The model under review builds one solid part; all positions refer to its coordinate system, in mm. A direction names the side the tool comes from. Round coordinates to 2 decimals unless told otherwise and drop trailing zeros. Order: outer loops, then holes, each group sorted by start corner. A loop starts at its lowest first (then second) coordinate and runs counter-clockwise, first axis right, second up.
```python
from build123d import *
from OCP.BRepFilletAPI import BRepFilletAPI_MakeChamfer

# Parameters (mm, degrees)
SKETCH3_R               = 27
BOSS_EXTRUDE1_DEPTH     = 6
BOSS_EXTRUDE2_DEPTH     = 126
SKETCH19_R              = 27
BOSS_EXTRUDE3_DEPTH     = 6
CUT_EXTRUDE5_REACH      = 139.412
SKETCH13_R              = 2.6
CUT_EXTRUDE6_REACH      = 145.185
SKETCH20_R              = 2.6
CUT_EXTRUDE7_REACH      = 145.185
SKETCH21_W              = 10
SKETCH21_H              = 41.952353926
RIB3_REACH              = 145.185
SKETCH18_WALL_W         = 329.601445786
SKETCH18_WALL_H         = 5
CIRPATTERN1_COUNT       = 3
MIRROR2_COPY_1_REACH    = 145.185
MIRROR2_COPY_1_SKETCH_W = 329.601445786
MIRROR2_COPY_1_SKETCH_H = 5
MIRROR2_COPY_2_REACH    = 145.185
MIRROR2_COPY_2_SKETCH_W = 329.601445786
MIRROR2_COPY_2_SKETCH_H = 5
FILLET1_R               = 12
CHAMFER1_SIZE           = 1
CHAMFER1_SIZE2          = 1.732050808
CHAMFER2_SIZE           = 1
CHAMFER3_SIZE           = 0.5


with BuildPart() as part:
    # Sketch3 → Boss-Extrude1 (new body)
    with BuildSketch(Plane(origin=(0, 0, 0), x_dir=(1, 0, 0), z_dir=(0, 1, 0))):
        with Locations(Location((0, 0, 0), (0, 0, 270))):
            Circle(SKETCH3_R)
    extrude(amount=BOSS_EXTRUDE1_DEPTH)

    # Sketch4 → Boss-Extrude2 (add)
    with BuildSketch(Plane(origin=(0, 6, 0), x_dir=(1, 0, 0), z_dir=(0, 1, 0))):
        Polygon((10, -5.773502692), (10, 5.773502692), (0, 11.547005384), (-10, 5.773502692), (-10, -5.773502692), (0, -11.547005384), align=None)
    extrude(amount=BOSS_EXTRUDE2_DEPTH)

    # Sketch19 → Boss-Extrude3 (add)
    with BuildSketch(Plane(origin=(0, 132, 0), x_dir=(1, 0, 0), z_dir=(0, 1, 0))):
        with Locations(Location((0, 0, 0), (0, 0, 270))):
            Circle(SKETCH19_R)
    extrude(amount=BOSS_EXTRUDE3_DEPTH)

    # Sketch13 → Cut-Extrude5 (cut, up to next)
    with BuildSketch(Plane(origin=(0, 6, 0), x_dir=(1, 0, 0), z_dir=(0, 1, 0)), mode=Mode.PRIVATE) as cut_extrude5_sk1:
        with Locations(Location((-19, 0, 0), (0, 0, 270))):
            Circle(SKETCH13_R)
    cut_extrude5_tool1 = extrude(cut_extrude5_sk1.sketch, amount=-CUT_EXTRUDE5_REACH, mode=Mode.PRIVATE) & part.part
    # Sketch13 → Cut-Extrude5 (cut, up to next)
    with BuildSketch(Plane(origin=(0, 6, 0), x_dir=(1, 0, 0), z_dir=(0, 1, 0)), mode=Mode.PRIVATE) as cut_extrude5_sk2:
        with Locations(Location((9.5, 16.454482672, 0), (0, 0, 270))):
            Circle(SKETCH13_R)
    cut_extrude5_tool2 = extrude(cut_extrude5_sk2.sketch, amount=-CUT_EXTRUDE5_REACH, mode=Mode.PRIVATE) & part.part
    # Sketch13 → Cut-Extrude5 (cut, up to next)
    with BuildSketch(Plane(origin=(0, 6, 0), x_dir=(1, 0, 0), z_dir=(0, 1, 0)), mode=Mode.PRIVATE) as cut_extrude5_sk3:
        with Locations(Location((9.5, -16.454482672, 0), (0, 0, 270))):
            Circle(SKETCH13_R)
    cut_extrude5_tool3 = extrude(cut_extrude5_sk3.sketch, amount=-CUT_EXTRUDE5_REACH, mode=Mode.PRIVATE) & part.part
    add(cut_extrude5_tool1.solids().sort_by_distance((-19, 6, 0))[0], mode=Mode.SUBTRACT)
    add(cut_extrude5_tool2.solids().sort_by_distance((9.5, 6, -16.454483))[0], mode=Mode.SUBTRACT)
    add(cut_extrude5_tool3.solids().sort_by_distance((9.5, 6, 16.454483))[0], mode=Mode.SUBTRACT)

    # Sketch20 → Cut-Extrude6 (cut, up to next)
    with BuildSketch(Plane(origin=(0, 138, 0), x_dir=(1, 0, 0), z_dir=(0, 1, 0)), mode=Mode.PRIVATE) as cut_extrude6_sk1:
        with Locations(Location((9.5, 16.454482672, 0), (0, 0, 270))):
            Circle(SKETCH20_R)
    cut_extrude6_tool1 = extrude(cut_extrude6_sk1.sketch, amount=-CUT_EXTRUDE6_REACH, mode=Mode.PRIVATE) & part.part
    # Sketch20 → Cut-Extrude6 (cut, up to next)
    with BuildSketch(Plane(origin=(0, 138, 0), x_dir=(1, 0, 0), z_dir=(0, 1, 0)), mode=Mode.PRIVATE) as cut_extrude6_sk2:
        with Locations(Location((9.5, -16.454482672, 0), (0, 0, 270))):
            Circle(SKETCH20_R)
    cut_extrude6_tool2 = extrude(cut_extrude6_sk2.sketch, amount=-CUT_EXTRUDE6_REACH, mode=Mode.PRIVATE) & part.part
    add(cut_extrude6_tool1.solids().sort_by_distance((9.5, 138, -16.454483))[0], mode=Mode.SUBTRACT)
    add(cut_extrude6_tool2.solids().sort_by_distance((9.5, 138, 16.454483))[0], mode=Mode.SUBTRACT)

    # Sketch21 → Cut-Extrude7 (cut, up to next)
    with BuildSketch(Plane(origin=(0, 138, 0), x_dir=(1, 0, 0), z_dir=(0, 1, 0)), mode=Mode.PRIVATE) as cut_extrude7_sk1:
        with Locations((-22, 0)):
            Rectangle(SKETCH21_W, SKETCH21_H)
    cut_extrude7_tool1 = extrude(cut_extrude7_sk1.sketch, amount=-CUT_EXTRUDE7_REACH, mode=Mode.PRIVATE) & part.part
    add(cut_extrude7_tool1.solids().sort_by_distance((-22, 138, 0))[0], mode=Mode.SUBTRACT)

    # Sketch18 wall → Rib3 (add, up to next)
    with BuildSketch(Plane(origin=(15, 26, 0), x_dir=(0.242535625036, -0.970142500145, 0), z_dir=(0.970142500145, 0.242535625036, 0)), mode=Mode.PRIVATE) as rib3_sk1:
        Rectangle(SKETCH18_WALL_W, SKETCH18_WALL_H)
    rib3_tool1 = extrude(rib3_sk1.sketch, amount=-RIB3_REACH, mode=Mode.PRIVATE) - part.part
    rib3 = rib3_tool1.solids().sort_by_distance((15, 26, 0))[0]
    add(rib3)

    # CirPattern1: Rib3 ×3 about axis
    cirpattern1_axis = Axis((0, 0, 0), (0, 1, 0))
    for i in range(1, CIRPATTERN1_COUNT):
        add(rib3.rotate(cirpattern1_axis, i * 360 / CIRPATTERN1_COUNT))

    # Mirror2: Rib3 across plane
    add(rib3.mirror(Plane.ZX.offset(69)))

    # Mirror2 copy 1 sketch → Mirror2 copy 1 (add, up to next)
    with BuildSketch(Plane(origin=(-7.5, 112, -12.990381057), x_dir=(-0.12126781251799995, 0.970142500145, -0.21004201260391314), z_dir=(-0.4850712500724998, -0.242535625036, -0.8401680504165185)), mode=Mode.PRIVATE) as mirror2_copy_1_sk1:
        Rectangle(MIRROR2_COPY_1_SKETCH_W, MIRROR2_COPY_1_SKETCH_H)
    mirror2_copy_1_tool1 = extrude(mirror2_copy_1_sk1.sketch, amount=-MIRROR2_COPY_1_REACH, mode=Mode.PRIVATE) - part.part
    add(mirror2_copy_1_tool1.solids().sort_by_distance((-7.5, 112, -12.990381057))[0])

    # Mirror2 copy 2 sketch → Mirror2 copy 2 (add, up to next)
    with BuildSketch(Plane(origin=(-7.5, 112, 12.990381057), x_dir=(-0.12126781251800012, 0.970142500145, 0.21004201260391306), z_dir=(-0.48507125007250046, -0.242535625036, 0.8401680504165182)), mode=Mode.PRIVATE) as mirror2_copy_2_sk1:
        Rectangle(MIRROR2_COPY_2_SKETCH_W, MIRROR2_COPY_2_SKETCH_H)
    mirror2_copy_2_tool1 = extrude(mirror2_copy_2_sk1.sketch, amount=-MIRROR2_COPY_2_REACH, mode=Mode.PRIVATE) - part.part
    add(mirror2_copy_2_tool1.solids().sort_by_distance((-7.5, 112, 12.990381057))[0])

    # Fillet1
    fillet1_edges = [part.edges().sort_by_distance(p)[0] for p in [
        (-17, 135, 20.976176963),
        (-17, 135, -20.976176963),
    ]]
    fillet(fillet1_edges, radius=FILLET1_R)

    # Chamfer1: one chamfer whose edges measure the first distance from different faces: ONE call of the kernel's chamfer builder (chamfer() names one face for all edges)
    chamfer1_edges_1 = [part.edges().sort_by_distance(p)[0] for p in [
        (10, 132, 4.136751346),
        (5, 132, -8.660254038),
        (-1.417468245, 132, -10.728629711),
        (-10, 132, 0),
        (-8.582531755, 132, 6.591878365),
        (10, 132, -4.136751346),
        (-1.417468245, 132, 10.728629711),
        (-8.582531755, 132, -6.591878365),
        (5, 132, 8.660254038),
    ]]
    chamfer1_side_1 = [part.faces().sort_by_distance(p)[0] for p in [
        (26.303437009, 132, 0),
    ]]
    chamfer1_edges_2 = [part.edges().sort_by_distance(p)[0] for p in [
        (-1.417468245, 6, 10.728629711),
        (-8.582531755, 6, -6.591878365),
        (10, 6, -4.136751346),
        (5, 6, 8.660254038),
        (10, 6, 4.136751346),
        (5, 6, -8.660254038),
        (-1.417468245, 6, -10.728629711),
        (-10, 6, 0),
        (-8.582531755, 6, 6.591878365),
    ]]
    chamfer1_side_2 = [part.faces().sort_by_distance(p)[0] for p in [
        (0, 6, -26.236324676),
    ]]
    chamfer1 = BRepFilletAPI_MakeChamfer(part.part.solid().wrapped)
    for e in chamfer1_edges_1:
        chamfer1.Add(CHAMFER1_SIZE, CHAMFER1_SIZE2, e.wrapped, chamfer1_side_1[0].wrapped)  # the first distance lies on this face
    for e in chamfer1_edges_2:
        chamfer1.Add(CHAMFER1_SIZE, CHAMFER1_SIZE2, e.wrapped, chamfer1_side_2[0].wrapped)  # the first distance lies on this face
    add(Compound.cast(chamfer1.Shape()), mode=Mode.REPLACE)

    # Chamfer2
    chamfer2_edges = [part.edges().sort_by_distance(p)[0] for p in [
        (0, 0, -27),
        (-17, 138, 0),
        (-17, 132, 0),
        (27, 132, 0),
        (-14.797958971, 132, 21.070338854),
        (-14.797958971, 132, -21.070338854),
        (27, 138, 0),
        (-14.797958971, 138, 21.070338854),
        (-14.797958971, 138, -21.070338854),
        (0, 6, -27),
    ]]
    chamfer(chamfer2_edges, length=CHAMFER2_SIZE)

    # Chamfer3
    chamfer3_edges = [part.edges().sort_by_distance(p)[0] for p in [
        (-19, 6, -2.6),
        (-19, 0, -2.6),
        (9.5, 6, -19.054482672),
        (9.5, 0, -19.054482672),
        (9.5, 6, 13.854482672),
        (9.5, 0, 13.854482672),
        (9.5, 132, -19.054482672),
        (9.5, 138, -19.054482672),
        (9.5, 132, 13.854482672),
        (9.5, 138, 13.854482672),
    ]]
    chamfer(chamfer3_edges, length=CHAMFER3_SIZE)


solid = part.part
```
(1) For faces 1 (the flat face through (13, 21, -2.5)), 2 (the flat face through (15, 132, 5)), 3 (the flat face through (-4.136, 20.976, 12.164)), 4 (the flat face through (13, 117, 2.5)), 5 (the flat face through (-9.1, 131.12, 6.86)), list the 3-axis set-ups (+Z, -Z, +X, -X, +Y, -Y) from which the entire face can be reached by the end or side of a thin tool; tool diameter is ignored.
Data:
face 1: -Z, +X
face 2: none
face 3: +Z
face 4: +Z, +X
face 5: -X
(2) Consider section B-B (y = 70). Write out the cut boundary in (x, z), and give its area (3 significant figures).
Data:
outline: (-10, -5.77) - (0, -11.55) - (10, -5.77) - (10, 5.77) - (0, 11.55) - (-10, 5.77) - close
area: 346 mm2
(3) Insertion check: pin 1 (12.5 mm diameter, centred on y = 76, z = 2.5, fed in from -X); pin 2 (4.5 mm diameter, centred on x = 9.5, z = -16.45, fed in from -Y); pin 3 (8 mm diameter, centred on y = 81, z = -12, fed in from -X); pin 4 (3 mm diameter, centred on x = 14.5, y = 120.5, fed in from -Z). Each pin has a flat end and moves straight along its axis. Give the tip position at first contact, or say it passes through.
Data:
pin 1: stops at x = -10
pin 2: passes through
pin 3: stops at x = -6.14
pin 4: stops at z = -2.5
(4) To check wall thickness, follow probe 1 along Y at (x, z) = (-14, 14); probe 2 along X at (y, z) = (2, 0); probe 3 along Z at (x, y) = (9, 2). State the ranges of each line that lie inside material, in increasing order.
Data:
probe 1: y = 0 to 6, 132 to 138
probe 2: x = -27 to -21.6, -16.4 to 27
probe 3: z = -25.46 to -19.01, -13.9 to 13.9, 19.01 to 25.46
(5) Draft analysis for pull direction X (two halves, no side actions). For faces 6 (the flat face through (5.323, 131.122, -9.043)), 7 (the flat face through (13, 21, 2.5)), 8 (the flat face through (-1.437, 131.122, 11.286)), state which applies: pulls with the +X half, pulls with the -X half, needs draft (parallel to the pull), parting line crosses it, or undercut.
Data:
face 6: pulls with the +X half
face 7: needs draft
face 8: undercut
